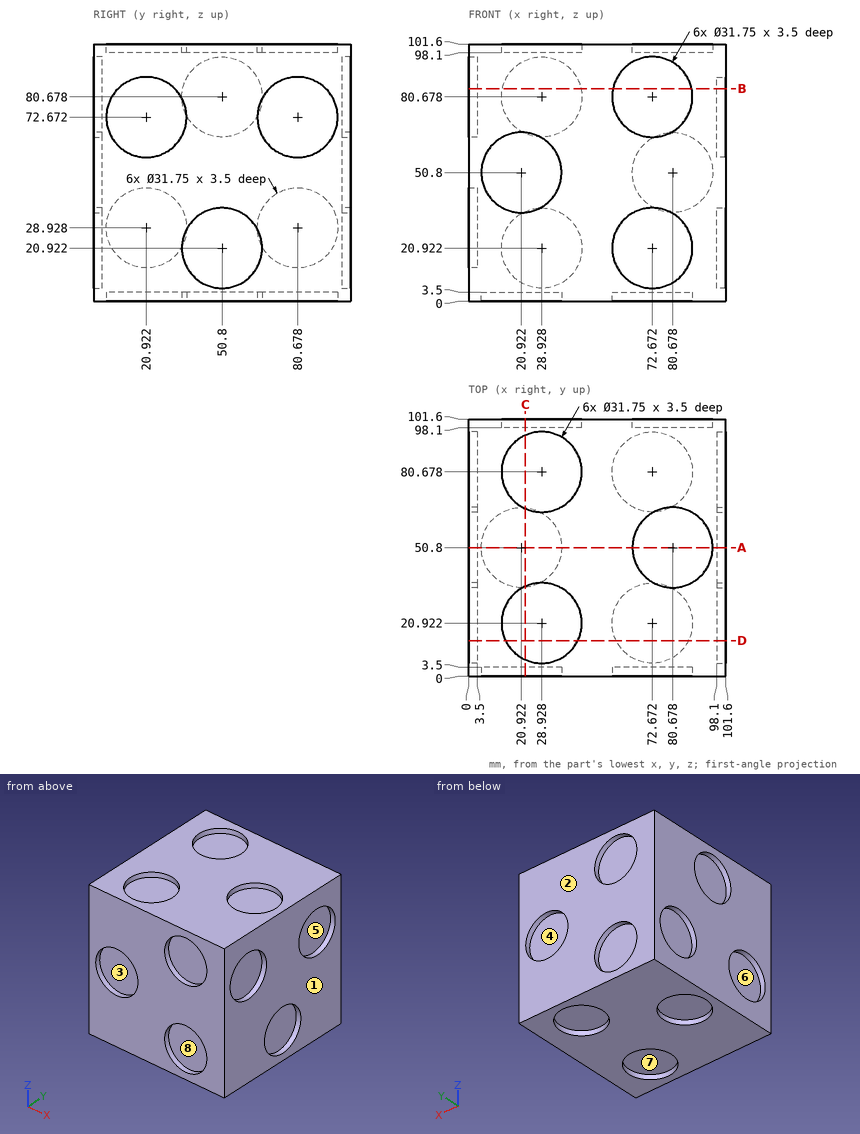
The drawing under review shows one solid part. Ordinate dimensions are in mm from its lowest x, y, z. A direction names the side the tool comes from. Coordinates: 2 decimals unless noted, no trailing zeros. Order: outer loops, then holes, each group sorted by start corner. A loop starts at its lowest first (then second) coordinate and runs counter-clockwise, first axis right, second up. Notation, with made-up numbers: (-23.75, 16) -> (12.25, 16) arc R12 ccw to (12.25, 33) -> close; hole circle Ø8 at (54.5, 79.5). An arc over 180 degrees is marked (long way). Return JSON: item names as keys, results as strings.
1. We need section D-D on y = 14. Write out the cut boundary in (x, z), and give its area (3 significant figures).
Answer block:
{"outline": "(0, 0) -> (58.39, 0) -> (58.39, 3.5) -> (86.96, 3.5) -> (86.96, 0) -> (101.6, 0) -> (101.6, 58.39) -> (98.1, 58.39) -> (98.1, 86.96) -> (101.6, 86.96) -> (101.6, 101.6) -> (43.21, 101.6) -> (43.21, 98.1) -> (14.64, 98.1) -> (14.64, 101.6) -> (0, 101.6) -> (0, 43.21) -> (3.5, 43.21) -> (3.5, 14.64) -> (0, 14.64) -> close", "area": "9,920 mm²"}
2. For line 1 (Z direction, x = 99, y = 50); line 2 (X direction, y = 50, z = 99); line 3 (Y direction, x = 15, z = 83.5), list the stretches that pass through material, from the lowest coordinate up. Write a range as from..to.
Answer block:
{"line 1": "0..5.07, 36.78..101.6", "line 2": "0..64.82, 96.53..101.6", "line 3": "0..98.1"}
3. Machinability: for the marked faces 5, 6, 7 and 8, which of the approach directions +Z, -Z, +X, -X, +Y, -Y give a long, thin tool a straight path to every point of the face, cutting with its end or side? Answer none if there is none.
Answer block:
{"face 5": "+X", "face 6": "-X", "face 7": "-Z", "face 8": "-Y"}
4. We need section B-B on z = 84. Write out the cut boundary in (x, y).
Answer block:
{"outline": "(0, 0) -> (57.15, 0) -> (57.15, 3.5) -> (88.2, 3.5) -> (88.2, 0) -> (101.6, 0) -> (101.6, 9.8) -> (98.1, 9.8) -> (98.1, 32.04) -> (101.6, 32.04) -> (101.6, 69.56) -> (98.1, 69.56) -> (98.1, 91.8) -> (101.6, 91.8) -> (101.6, 101.6) -> (44.45, 101.6) -> (44.45, 98.1) -> (13.4, 98.1) -> (13.4, 101.6) -> (0, 101.6) -> (0, 66.32) -> (3.5, 66.32) -> (3.5, 35.28) -> (0, 35.28) -> close"}
5. The part is to be moulded in two halves that separate along X. For the marked faces 1, 2, 3 and 4, say which applies: +X half, -X half, draft (parallel to the pull), parting line (faces both ways), or undercut.
Answer block:
{"face 1": "+X half", "face 2": "draft", "face 3": "undercut", "face 4": "undercut"}
6. We need section C-C on x = 22.5. Write out the cut boundary in (y, z), and give its area (4 significant figures).
Answer block:
{"outline": "(0, 0) -> (35, 0) -> (35, 3.5) -> (66.6, 3.5) -> (66.6, 0) -> (101.6, 0) -> (101.6, 6.41) -> (98.1, 6.41) -> (98.1, 35.44) -> (101.6, 35.44) -> (101.6, 66.16) -> (98.1, 66.16) -> (98.1, 95.19) -> (101.6, 95.19) -> (101.6, 101.6) -> (95.19, 101.6) -> (95.19, 98.1) -> (66.16, 98.1) -> (66.16, 101.6) -> (35.44, 101.6) -> (35.44, 98.1) -> (6.41, 98.1) -> (6.41, 101.6) -> (0, 101.6) -> (0, 66.6) -> (3.5, 66.6) -> (3.5, 35) -> (0, 35) -> close", "area": "9,695 mm²"}
7. We need section A-A on y = 50.8. Write out the cut boundary in (x, z).
Answer block:
{"outline": "(0, 0) -> (5.05, 0) -> (5.05, 3.5) -> (36.8, 3.5) -> (36.8, 0) -> (101.6, 0) -> (101.6, 5.05) -> (98.1, 5.05) -> (98.1, 36.8) -> (101.6, 36.8) -> (101.6, 101.6) -> (96.55, 101.6) -> (96.55, 98.1) -> (64.8, 98.1) -> (64.8, 101.6) -> (0, 101.6) -> (0, 96.55) -> (3.5, 96.55) -> (3.5, 64.8) -> (0, 64.8) -> close"}
8. For pin 1 Ø16 at (x, y) = (68.5, 86) entering from -Z; pin 2 Ø10 at (y, z) = (78.5, 34) entering from -X; pin 3 Ø16 at (x, z) = (66, 80) entering from -Y, all flat-tipped, find the tip position at first contact; note any pin that passes through.
Answer block:
{"pin 1": "z = 3.5", "pin 2": "x = 3.5", "pin 3": "y = 3.5"}
